Here's how the part is built. I have some questions about the finished solid (model axes, mm). Coordinates: 2 decimals unless noted, no trailing zeros. Write each loop counter-clockwise with the first axis right and the second up, starting at its lowest first coordinate (ties: lowest second). Pieces come first, ordered by that corner, then holes.
Item 1: Please list where these lines run through material, in increasing order: line 1 (Z direction, x = -68.5, y = 1.45); line 2 (X direction, y = 2.45, z = -9); line 3 (Z direction, x = 31.5, y = 0.75).
Item 2: I'm going to push flat-ended pins straight in: P1, Ø12, axis at x = 55, z = -2, coming from the -Y side; P2, Ø4, axis at x = 9, z = 54.5, coming from the +Y side (3 decimals). Where does each tip first touch, or does it pass through?
Item 3: I want a section at D-D (z = -9.5). Please give me the cut outline in (x, y) (1 decimal), and give its area (3 significant figures).
Item 4: I want a section at C-C (y = 1.2). Count the separate pieces of the cut face and the enclosed holes in it, and give its area (3 significant figures).
Item 5: I want a section at A-A (z = 38). Please give me the cut outline in (x, y) (3 decimals), and give its area (3 significant figures).
Item 6: If we mould it in two halves opening along Z, with no side actions, what happens to faces 1 (the face through (-76.5, 2, 1)), 2 (the face through (15.335, 1.61, 0.078)), 3 (the face through (-1, 2, 63.5)), 4 (the face through (-1, 2, -63.5))? For each: pulls with the +Z half, pulls with the -Z half, needs draft (parallel to the pull), parting line crosses it, or undercut.
Item 7: I want a section at B-B (x = -45). Please give me the cut outline in (y, z) (3 decimals).
from build123d import *

# Parameters (mm, degrees)
SKETCH1_W             = 153
SKETCH1_H             = 127.000000028
BOSS_EXTRUDE1_DEPTH   = 3.175
M3X0_5_TAPPED_HOLE1_D = 2.5
SKETCH4_R             = 2.75
CUT_EXTRUDE1_DEPTH    = 4.175
CUT_EXTRUDE2_DEPTH    = 4.175


with BuildPart() as part:
    # Sketch1 → Boss-Extrude1 (new body)
    with BuildSketch(Plane(origin=(0, 0, 0), x_dir=(1, 0, 0), z_dir=(0, 1, 0))):
        Rectangle(SKETCH1_W, SKETCH1_H)
    extrude(amount=BOSS_EXTRUDE1_DEPTH)

    # M3x0.5 Tapped Hole1 (through all)
    with Locations(Plane(origin=(0, 3.175, 0), x_dir=(-1, 0, 0), z_dir=(0, 1, 0))):
        with Locations((62, -54.500000014), (38, -54.500000014), (9, -54.500000014), (-9, -54.500000014), (-38, -54.500000014), (-62, -54.500000014), (-62, 54.500000014), (-38, 54.500000014), (-9, 54.500000014), (9, 54.500000014), (38, 54.500000014), (62, 54.500000014), (-31.5, 54.500000014), (-68.5, 54.500000014), (-68.5, -54.500000014), (-31.5, -54.500000014), (31.5, -54.500000014), (68.5, -54.500000014), (31.5, 54.500000014), (68.5, 54.500000014)):
            Hole(M3X0_5_TAPPED_HOLE1_D / 2)

    # Sketch4 → Cut-Extrude1 (cut, through all)
    with BuildSketch(Plane(origin=(0, 3.175, 0), x_dir=(1, 0, 0), z_dir=(0, 1, 0))):
        with Locations(Location((-70, 38, 0), (0, 0, 270))):  # turned: the seam where the file's is
            Circle(SKETCH4_R)
        with Locations(Location((-70, -38, 0), (0, 0, 270))):  # turned: the seam where the file's is
            Circle(SKETCH4_R)
        with Locations(Location((70, -38, 0), (0, 0, 270))):  # turned: the seam where the file's is
            Circle(SKETCH4_R)
        with Locations(Location((70, 38, 0), (0, 0, 270))):  # turned: the seam where the file's is
            Circle(SKETCH4_R)
    extrude(amount=-CUT_EXTRUDE1_DEPTH, mode=Mode.SUBTRACT)

    # Sketch5 → Cut-Extrude2 (cut, through all)
    with BuildSketch(Plane(origin=(0, 3.175, 0), x_dir=(1, 0, 0), z_dir=(0, 1, 0))):
        with BuildLine():
            Line((-23.070812682, 43.500000014), (23.070812682, 43.500000014))
            ThreePointArc((23.070812682, 43.500000014), (29.043622339, 39.30593248), (27.126552604, 32.263951132))
            Line((27.126552604, 32.263951132), (4.055739923, 13.113668706))
            ThreePointArc((4.055739923, 13.113668706), (0, 11.649717588), (-4.055739923, 13.113668706))
            Line((-4.055739923, 13.113668706), (-27.126552604, 32.263951132))
            ThreePointArc((-27.126552604, 32.263951132), (-29.043622339, 39.30593248), (-23.070812682, 43.500000014))
        make_face()
        with BuildLine():
            Line((-61.5, 27.778386997), (-61.5, -27.778386997))
            ThreePointArc((-61.5, -27.778386997), (-57.848939745, -33.526275675), (-51.094260077, -32.66443588))
            Line((-51.094260077, -32.66443588), (-17.628959214, -4.886048882))
            ThreePointArc((-17.628959214, -4.886048882), (-15.334699136, 0), (-17.628959214, 4.886048882))
            Line((-17.628959214, 4.886048882), (-51.094260077, 32.66443588))
            ThreePointArc((-51.094260077, 32.66443588), (-57.848939745, 33.526275675), (-61.5, 27.778386997))
        make_face()
        with BuildLine():
            Line((4.055739923, -13.113668706), (27.126552604, -32.263951132))
            ThreePointArc((27.126552604, -32.263951132), (29.043622339, -39.30593248), (23.070812682, -43.500000014))
            Line((23.070812682, -43.500000014), (-23.070812682, -43.500000014))
            ThreePointArc((-23.070812682, -43.500000014), (-29.043622339, -39.30593248), (-27.126552604, -32.263951132))
            Line((-27.126552604, -32.263951132), (-4.055739923, -13.113668706))
            ThreePointArc((-4.055739923, -13.113668706), (0, -11.649717588), (4.055739923, -13.113668706))
        make_face()
        with BuildLine():
            Line((61.5, 27.778386997), (61.5, -27.778386997))
            ThreePointArc((61.5, -27.778386997), (57.848939745, -33.526275675), (51.094260077, -32.66443588))
            Line((51.094260077, -32.66443588), (17.628959214, -4.886048882))
            ThreePointArc((17.628959214, -4.886048882), (15.334699136, 0), (17.628959214, 4.886048882))
            Line((17.628959214, 4.886048882), (51.094260077, 32.66443588))
            ThreePointArc((51.094260077, 32.66443588), (57.848939745, 33.526275675), (61.5, 27.778386997))
        make_face()
    extrude(amount=-CUT_EXTRUDE2_DEPTH, mode=Mode.SUBTRACT)


solid = part.part
Answer:
1. line 1: z = -63.5 to -55.75, -53.25 to -40.3, -35.7 to 35.7, 40.3 to 53.25, 55.75 to 63.5
1. line 2: x = -76.5 to -61.5, -22.59 to 22.59, 61.5 to 76.5
1. line 3: z = -63.5 to -55.75, -53.25 to -16.4, 16.4 to 53.25, 55.75 to 63.5
2. P1: passes through
2. P2: stops at y = 3.175
3. outline: (-76.5, 0) - (-61.5, 0) - (-61.5, 3.2) - (-76.5, 3.2) - close; (-23.2, 0) - (23.2, 0) - (23.2, 3.2) - (-23.2, 3.2) - close; (61.5, 0) - (76.5, 0) - (76.5, 3.2) - (61.5, 3.2) - close
3. area: 242 mm2
4. separate pieces: 1
4. enclosed holes: 28
4. area: 12,800 mm2
5. outline: (-76.5, 0) - (-72.75, 0) - (-72.75, 3.175) - (-76.5, 3.175) - close; (-67.25, 0) - (-29.364, 0) - (-29.364, 3.175) - (-67.25, 3.175) - close; (29.364, 0) - (67.25, 0) - (67.25, 3.175) - (29.364, 3.175) - close; (72.75, 0) - (76.5, 0) - (76.5, 3.175) - (72.75, 3.175) - close
5. area: 264 mm2
6. face 1: needs draft
6. face 2: undercut
6. face 3: pulls with the +Z half
6. face 4: pulls with the -Z half
7. outline: (0, -63.5) - (3.175, -63.5) - (3.175, -27.606) - (0, -27.606) - close; (0, 27.606) - (3.175, 27.606) - (3.175, 63.5) - (0, 63.5) - close
